Autodesk Inventor part; units mm, degrees
ref_plane "YZ Plane" through (0, 0, 0) normal (1, 0, 0) x (0, 1, 0)
ref_plane "XZ Plane" through (0, 0, 0) normal (0, 1, 0) x (-1, 0, 0)
ref_plane "XY Plane" through (0, 0, 0) normal (0, 0, 1) x (1, 0, 0)
sketch "Sketch1" plane through (0, 0, 0) normal (0, 0, 1) x (1, 0, 0)
  line L0 (0, 0) -> (44, 0)
  line L1 (44, 0) -> (44, 44)
  line L2 (44, 44) -> (0, 44)
  line L3 (0, 44) -> (0, 0)
  dimension "d5" = 44
  dimension "d6" = 44
extrude "JOKAB, 44MM" add sketch "Sketch1" along normal blind 100
sketch "Sketch2" plane through (0, 0, 100) normal (0, 0, 1) x (1, 0, 0)
  line L0 (44, 0) -> (0, 0)
  line L1 (0, 44) -> (44, 44)
  line L2 (44, 44) -> (0, 44)
  line L3 (16.5, 44) -> (16.5, 40.7)
  line L4 (11.875, 40.7) -> (11.875, 37.9667)
  line L5 (11.875, 37.9667) -> (17.3417, 32.5)
  line L6 (22, 44) -> (22, 0) construction
  line L7 (0, 44) -> (0, 0)
  line L8 (0, 22) -> (44, 22) construction
  line L9 (44, 0) -> (44, 44)
  line L10 (17.3417, 32.5) -> (22, 32.5)
  line L11 (11.875, 40.7) -> (16.5, 40.7)
  line L12 (27.5, 44) -> (27.5, 40.7)
  line L13 (32.125, 40.7) -> (32.125, 37.9667)
  line L14 (32.125, 37.9667) -> (26.6583, 32.5)
  line L15 (26.6583, 32.5) -> (22, 32.5)
  line L16 (32.125, 40.7) -> (27.5, 40.7)
  line L17 (16.5, 0) -> (16.5, 3.3)
  line L18 (11.875, 3.3) -> (11.875, 6.0333)
  line L19 (11.875, 6.0333) -> (17.3417, 11.5)
  line L20 (17.3417, 11.5) -> (22, 11.5)
  line L21 (11.875, 3.3) -> (16.5, 3.3)
  line L22 (27.5, 0) -> (27.5, 3.3)
  line L23 (32.125, 3.3) -> (27.5, 3.3)
  line L24 (32.125, 3.3) -> (32.125, 6.0333)
  line L25 (32.125, 6.0333) -> (26.6583, 11.5)
  line L26 (26.6583, 11.5) -> (22, 11.5)
  line L27 (0, 16.5) -> (3.3, 16.5)
  line L28 (3.3, 11.875) -> (6.0333, 11.875)
  line L29 (6.0333, 11.875) -> (11.5, 17.3417)
  line L30 (22, 0) -> (22, 44) construction
  line L31 (11.5, 17.3417) -> (11.5, 22)
  line L32 (3.3, 11.875) -> (3.3, 16.5)
  line L33 (0, 27.5) -> (3.3, 27.5)
  line L34 (3.3, 32.125) -> (3.3, 27.5)
  line L35 (3.3, 32.125) -> (6.0333, 32.125)
  line L36 (6.0333, 32.125) -> (11.5, 26.6583)
  line L37 (11.5, 26.6583) -> (11.5, 22)
  line L38 (27.5, 0) -> (27.5, 3.3)
  line L39 (32.125, 3.3) -> (32.125, 6.0333)
  line L40 (32.125, 6.0333) -> (26.6583, 11.5)
  line L41 (44, 22) -> (0, 22) construction
  line L42 (26.6583, 11.5) -> (22, 11.5)
  line L43 (32.125, 3.3) -> (27.5, 3.3)
  line L44 (16.5, 0) -> (16.5, 3.3)
  line L45 (11.875, 3.3) -> (16.5, 3.3)
  line L46 (11.875, 3.3) -> (11.875, 6.0333)
  line L47 (11.875, 6.0333) -> (17.3417, 11.5)
  line L48 (17.3417, 11.5) -> (22, 11.5)
  line L49 (44, 27.5) -> (40.7, 27.5)
  line L50 (40.7, 32.125) -> (37.9667, 32.125)
  line L51 (37.9667, 32.125) -> (32.5, 26.6583)
  line L52 (22, 44) -> (22, 0) construction
  line L53 (32.5, 26.6583) -> (32.5, 22)
  line L54 (40.7, 32.125) -> (40.7, 27.5)
  line L55 (44, 16.5) -> (40.7, 16.5)
  line L56 (40.7, 11.875) -> (40.7, 16.5)
  line L57 (40.7, 11.875) -> (37.9667, 11.875)
  line L58 (37.9667, 11.875) -> (32.5, 17.3417)
  line L59 (32.5, 17.3417) -> (32.5, 22)
  line L60 (27.5, 44) -> (16.5, 44)
  line L61 (44, 27.5) -> (44, 16.5)
  line L62 (27.5, 0) -> (16.5, 0)
  line L63 (0, 16.5) -> (0, 27.5)
  point P0 (22, 22)
  point P1 (22, 22)
  point P2 (22, 22)
  point P3 (22, 22)
  dimension "d10" = 5.5
  dimension "d11" = 10.125
  dimension "d12" = 11.5
  dimension "d13" = 45
  dimension "d15" = 2.7333
  dimension "d17" = 8.2
  dimension "d20" = 360
extrude "Extrusion2" cut sketch "Sketch2" against normal through all contours L0 L17 L21 L18 L19 L20 L26 L25 L24 L23 L22 | L55 L56 L57 L58 L59 L53 L51 L50 L54 L49 L9 | L7 L33 L34 L35 L36 L37 L31 L29 L28 L32 L27 | L12 L16 L13 L14 L15 L10 L5 L4 L11 L3 L1
sketch "Sketch3" plane through (0, 0, 100) normal (0, 0, 1) x (1, 0, 0)
  line L0 (11.5, 26.6583) -> (11.5, 17.3417)
  line L1 (17.3417, 11.5) -> (26.6583, 11.5)
  line L2 (32.5, 17.3417) -> (32.5, 26.6583)
  line L3 (26.6583, 32.5) -> (17.3417, 32.5)
  line L4 (13.2688, 13.2687) -> (13.2687, 30.7313)
  line L5 (13.2687, 30.7313) -> (30.7312, 30.7313)
  line L6 (30.7312, 30.7313) -> (30.7313, 13.2688)
  line L7 (30.7313, 13.2688) -> (13.2688, 13.2687)
  line L8 (32.5, 22) -> (11.5, 22) construction
  line L9 (22, 32.5) -> (22, 11.5) construction
  dimension "d36" = 17.4625
  dimension "d37" = 8.7312
  dimension "d38" = 17.4625
  dimension "d39" = 8.7312
extrude "Extrusion3" cut sketch "Sketch3" against normal through all
sketch "Sketch4" plane through (0, 0, 100) normal (0, 0, 1) x (1, 0, 0)
  line L0 (11.5, 26.6583) -> (11.5, 17.3417)
  line L1 (17.3417, 11.5) -> (26.6583, 11.5)
  line L2 (32.5, 17.3417) -> (32.5, 26.6583)
  line L3 (44, 44) -> (44, 27.5)
  line L4 (27.5, 44) -> (44, 44)
  line L5 (26.6583, 32.5) -> (17.3417, 32.5)
  line L6 (40.7, 32.7625) -> (32.7625, 32.7625)
  line L7 (32.7625, 32.7625) -> (32.7625, 40.7)
  line L8 (32.7625, 40.7) -> (40.7, 40.7)
  line L9 (40.7, 40.7) -> (40.7, 32.7625)
  line L10 (32.5, 22) -> (11.5, 22)
  line L11 (22, 32.5) -> (22, 11.5)
  line L12 (3.3, 32.7625) -> (11.2375, 32.7625)
  line L13 (11.2375, 32.7625) -> (11.2375, 40.7)
  line L14 (11.2375, 40.7) -> (3.3, 40.7)
  line L15 (3.3, 40.7) -> (3.3, 32.7625)
  line L16 (40.7, 11.2375) -> (32.7625, 11.2375)
  line L17 (32.7625, 11.2375) -> (32.7625, 3.3)
  line L18 (32.7625, 3.3) -> (40.7, 3.3)
  line L19 (40.7, 3.3) -> (40.7, 11.2375)
  line L20 (11.2375, 11.2375) -> (11.2375, 3.3)
  line L21 (11.2375, 3.3) -> (3.3, 3.3)
  line L22 (3.3, 3.3) -> (3.3, 11.2375)
  line L23 (3.3, 11.2375) -> (11.2375, 11.2375)
  dimension "d30" = 3.3
  dimension "d31" = 3.3
  dimension "d32" = 7.9375
  dimension "d33" = 7.9375
extrude "Extrusion4" cut sketch "Sketch4" against normal through all
equation "\"d15\" = 0.333333 * d17"
equation "\"d37\" = 0.5 * d36"
equation "\"d38\" = d36"
equation "\"d39\" = d37"
equation "\"d31\" = d30"
equation "\"d33\" = d32"
properties part number "BAR, EXTRUDED, ALUM, 44MMX44MM, JOKAB" material "Aluminum, 6061"
Source: CAD feature listing. Evaluate the final solid. Frame: model axes, mm. A direction names the side the tool comes from. Coordinates: 2 decimals unless noted, no trailing zeros. Loops run counter-clockwise (first coordinate to the right, second up) from the corner with the lowest first, then second, coordinate; pieces in that order, holes last. Notation, with made-up numbers: (39.5, -5.75) - (45.5, -5.75) arc R27 ccw to (45.5, 26.25) - close; hole circle Ø7 at (-30, 38). An arc over 180 degrees is marked (long way). Return JSON: item names as keys, results as strings.
Q1. Material intervals for line 1 along X through (y, z) = (4, 76.5) (1 decimal); line 2 along Y through (x, z) = (21, 73), sorted ascending.
Results:
{"line 1": "0 to 3.3, 11.2 to 11.9, 32.1 to 32.8, 40.7 to 44", "line 2": "11.5 to 13.27, 30.73 to 32.5"}
Q2. Mould query, pull axis Y, two halves, no side actions, for faces 1 (the flat face through (30, 3.3, 51)), 2 (the flat face through (12, 22, 100)). Classes: released by +Y, released by -Y, zero draft, split by the parting line, or undercut.
Results:
{"face 1": "undercut", "face 2": "zero draft"}
Q3. Section B-B, the plane x = 15.5. Return loops of the section in (y, z), plus the area to 3 significant figures.
Results:
{"outline": "(0, 0) - (3.3, 0) - (3.3, 100) - (0, 100) - close; (9.66, 0) - (13.27, 0) - (13.27, 100) - (9.66, 100) - close; (30.73, 0) - (34.34, 0) - (34.34, 100) - (30.73, 100) - close; (40.7, 0) - (44, 0) - (44, 100) - (40.7, 100) - close", "area": "1,380 mm2"}
Q4. Access query for faces 3 (the flat face through (7, 32.763, 51)), 4 (the flat face through (44, 36, 49)), 5 (the flat face through (27.5, 42, 51)), 6 (the flat face through (42, 16.5, 51)), 7 (the flat face through (2, 16.5, 51)). Directions: +Z, -Z, +X, -X, +Y, -Y. A direction counts if a zero-diameter tool reaches every point of the face in a straight line with its end or side. Return the directions, or none.
Results:
{"face 3": "+Z, -Z", "face 4": "+Z, -Z, +X, +Y, -Y", "face 5": "+Z, -Z, +Y", "face 6": "+Z, -Z, +X", "face 7": "+Z, -Z, -X"}
Q5. Section C-C, the plane x = 20. Return loops of the section in (y, z).
Results:
{"outline": "(11.5, 0) - (13.27, 0) - (13.27, 100) - (11.5, 100) - close; (30.73, 0) - (32.5, 0) - (32.5, 100) - (30.73, 100) - close"}
Q6. Contact query for flat-ended pins moving along their axis: P1, Ø1, axis at x = 20, z = 11.5, coming from the +Y side; P2, Ø6, axis at y = 22.5, z = 73, coming from the +X side. Output: stop coordinate, or through.
Results:
{"P1": "y = 32.5", "P2": "x = 32.5"}
Q7. Section D-D, the plane z = 40.5. Give the number of separate pieces and of enclosed holes in the cut face, plus the area to 3 significant figures.
Results:
{"separate pieces": "1", "enclosed holes": "5", "area": "689 mm2"}
Q8. Section A-A, the plane y = 39.5. Return loops of the section in (x, z) (1 decimal).
Results:
{"outline": "(0, 0) - (3.3, 0) - (3.3, 100) - (0, 100) - close; (11.2, 0) - (11.9, 0) - (11.9, 100) - (11.2, 100) - close; (32.1, 0) - (32.8, 0) - (32.8, 100) - (32.1, 100) - close; (40.7, 0) - (44, 0) - (44, 100) - (40.7, 100) - close"}
